```python
from build123d import *

# Parameters (mm, degrees)
F0_R         = 11.43
F0_R_2       = 14.605
F1_DEPTH     = 3.4925
F2_T1_DEPTH  = 15.875
F2_T3_DEPTH  = 15.875
F2_T5_DEPTH  = 15.875
F2_T7_DEPTH  = 15.875
F2_T10_ANGLE = 180
F2_T12_ANGLE = 90
F2_T14_ANGLE = 180
F2_T16_ANGLE = 90
F2_T18_ANGLE = 180
F2_T20_ANGLE = 90
F2_T22_ANGLE = 180
F2_T24_ANGLE = 90


# Not quite as in the source:
# - a fillet or chamfer that OpenCascade refuses, or shapes differently, is made with other operations: its cross-section is extruded or revolved along the edge and cut away or added


with BuildPart() as f1:
    # F0 (on Top) → F1 (new body)
    with BuildSketch(Plane.XY):
        with BuildLine():
            ThreePointArc((-14.605, 38.1), (0, 23.495), (14.605, 38.1))
            ThreePointArc((14.605, 38.1), (0, 52.705), (-14.605, 38.1))
        make_face()
        with Locations((0, 38.1)):
            Circle(F0_R, mode=Mode.SUBTRACT)
        with BuildLine():
            Line((14.605, 22.225), (14.605, 38.1))
            ThreePointArc((14.605, 38.1), (0, 23.495), (-14.605, 38.1))
            Line((-14.605, 38.1), (-14.605, 22.225))
            ThreePointArc((-14.605, 22.225), (-16.8368463274, 16.8368463274), (-22.225, 14.605))
            Line((-22.225, 14.605), (-38.1, 14.605))
            ThreePointArc((-38.1, 14.605), (-27.7727054608, 10.3272945392), (-23.495, 0))
            ThreePointArc((-23.495, 0), (-27.7727054608, -10.3272945392), (-38.1, -14.605))
            Line((-38.1, -14.605), (-22.225, -14.605))
            ThreePointArc((-22.225, -14.605), (-16.8368463274, -16.8368463274), (-14.605, -22.225))
            Line((-14.605, -22.225), (-14.605, -38.1))
            ThreePointArc((-14.605, -38.1), (0, -23.495), (14.605, -38.1))
            Line((14.605, -38.1), (14.605, -22.225))
            ThreePointArc((14.605, -22.225), (16.8368463274, -16.8368463274), (22.225, -14.605))
            Line((22.225, -14.605), (38.1, -14.605))
            ThreePointArc((38.1, -14.605), (23.495, 0), (38.1, 14.605))
            Line((38.1, 14.605), (22.225, 14.605))
            ThreePointArc((22.225, 14.605), (16.8368463274, 16.8368463274), (14.605, 22.225))
        make_face()
        Circle(F0_R_2, mode=Mode.SUBTRACT)
        with BuildLine():
            ThreePointArc((52.705, 0), (48.4272945392, 10.3272945392), (38.1, 14.605))
            ThreePointArc((38.1, 14.605), (23.495, 0), (38.1, -14.605))
            ThreePointArc((38.1, -14.605), (48.4272945392, -10.3272945392), (52.705, 0))
        make_face()
        with Locations((38.1, 0)):
            Circle(F0_R, mode=Mode.SUBTRACT)
        with BuildLine():
            ThreePointArc((-23.495, 0), (-27.7727054608, 10.3272945392), (-38.1, 14.605))
            ThreePointArc((-38.1, 14.605), (-52.705, 0), (-38.1, -14.605))
            ThreePointArc((-38.1, -14.605), (-27.7727054608, -10.3272945392), (-23.495, 0))
        make_face()
        with Locations((-38.1, 0)):
            Circle(F0_R, mode=Mode.SUBTRACT)
        with BuildLine():
            ThreePointArc((-14.605, -38.1), (0, -52.705), (14.605, -38.1))
            ThreePointArc((14.605, -38.1), (0, -23.495), (-14.605, -38.1))
        make_face()
        with Locations((0, -38.1)):
            Circle(F0_R, mode=Mode.SUBTRACT)
        Circle(F0_R_2)
        Circle(F0_R, mode=Mode.SUBTRACT)
    extrude(amount=F1_DEPTH)

    # F2: fillet of radius 5.08 on 1 edges, made by hand

    # F2_s2 → F2_t1 (cut)
    with BuildSketch(Plane.XZ.offset(22.225)):
        with BuildLine():
            ThreePointArc((-14.605, 0), (-12.7578317887, 2.5277703435), (-9.7794177812, 3.4925))
            Line((-9.7794177812, 3.4925), (-14.605, 3.4925))
            Line((-14.605, 3.4925), (-14.605, 0))
        make_face()
        with BuildLine():
            ThreePointArc((14.605, 0), (12.7578317887, 2.5277703435), (9.7794177812, 3.4925))
            Line((9.7794177812, 3.4925), (14.605, 3.4925))
            Line((14.605, 3.4925), (14.605, 0))
        make_face()
    extrude(amount=F2_T1_DEPTH, mode=Mode.SUBTRACT)

    # F2_s4 → F2_t3 (cut)
    with BuildSketch(Plane.YZ.offset(22.225)):
        with BuildLine():
            ThreePointArc((-14.605, 0), (-12.7578317887, 2.5277703435), (-9.7794177812, 3.4925))
            Line((-9.7794177812, 3.4925), (-14.605, 3.4925))
            Line((-14.605, 3.4925), (-14.605, 0))
        make_face()
        with BuildLine():
            ThreePointArc((14.605, 0), (12.7578317887, 2.5277703435), (9.7794177812, 3.4925))
            Line((9.7794177812, 3.4925), (14.605, 3.4925))
            Line((14.605, 3.4925), (14.605, 0))
        make_face()
    extrude(amount=F2_T3_DEPTH, mode=Mode.SUBTRACT)

    # F2_s6 → F2_t5 (cut)
    with BuildSketch(Plane.XZ.offset(-38.1)):
        with BuildLine():
            ThreePointArc((14.605, 0), (12.7578317887, 2.5277703435), (9.7794177812, 3.4925))
            Line((9.7794177812, 3.4925), (14.605, 3.4925))
            Line((14.605, 3.4925), (14.605, 0))
        make_face()
        with BuildLine():
            ThreePointArc((-14.605, 0), (-12.7578317887, 2.5277703435), (-9.7794177812, 3.4925))
            Line((-9.7794177812, 3.4925), (-14.605, 3.4925))
            Line((-14.605, 3.4925), (-14.605, 0))
        make_face()
    extrude(amount=F2_T5_DEPTH, mode=Mode.SUBTRACT)

    # F2_s8 → F2_t7 (cut)
    with BuildSketch(Plane.YZ.offset(-38.1)):
        with BuildLine():
            ThreePointArc((14.605, 0), (12.7578317887, 2.5277703435), (9.7794177812, 3.4925))
            Line((9.7794177812, 3.4925), (14.605, 3.4925))
            Line((14.605, 3.4925), (14.605, 0))
        make_face()
        with BuildLine():
            ThreePointArc((-14.605, 0), (-12.7578317887, 2.5277703435), (-9.7794177812, 3.4925))
            Line((-9.7794177812, 3.4925), (-14.605, 3.4925))
            Line((-14.605, 3.4925), (-14.605, 0))
        make_face()
    extrude(amount=F2_T7_DEPTH, mode=Mode.SUBTRACT)

    # F2_s9 → F2_t10 (revolve, cut)
    with BuildSketch(Plane.XZ.offset(38.1)):
        with BuildLine():
            ThreePointArc((-14.605, 0), (-12.7578317887, 2.5277703435), (-9.7794177812, 3.4925))
            Line((-9.7794177812, 3.4925), (-14.605, 3.4925))
            Line((-14.605, 3.4925), (-14.605, 0))
        make_face()
    revolve(axis=Axis((0, -38.1, 3.4925), (0, 0, 1)), revolution_arc=F2_T10_ANGLE, mode=Mode.SUBTRACT)

    # F2_s11 → F2_t12 (revolve, cut)
    with BuildSketch(Plane.XZ.offset(22.225)):
        with BuildLine():
            ThreePointArc((14.605, 0), (12.7578317887, 2.5277703435), (9.7794177812, 3.4925))
            Line((9.7794177812, 3.4925), (14.605, 3.4925))
            Line((14.605, 3.4925), (14.605, 0))
        make_face()
    revolve(axis=Axis((22.225, -22.225, 3.4925), (0, 0, -1)), revolution_arc=F2_T12_ANGLE, mode=Mode.SUBTRACT)

    # F2_s13 → F2_t14 (revolve, cut)
    with BuildSketch(Plane.YZ.offset(38.1)):
        with BuildLine():
            ThreePointArc((-14.605, 0), (-12.7578317887, 2.5277703435), (-9.7794177812, 3.4925))
            Line((-9.7794177812, 3.4925), (-14.605, 3.4925))
            Line((-14.605, 3.4925), (-14.605, 0))
        make_face()
    revolve(axis=Axis((38.1, 0, 3.4925), (0, 0, 1)), revolution_arc=F2_T14_ANGLE, mode=Mode.SUBTRACT)

    # F2_s15 → F2_t16 (revolve, cut)
    with BuildSketch(Plane.YZ.offset(22.225)):
        with BuildLine():
            ThreePointArc((14.605, 0), (12.7578317887, 2.5277703435), (9.7794177812, 3.4925))
            Line((9.7794177812, 3.4925), (14.605, 3.4925))
            Line((14.605, 3.4925), (14.605, 0))
        make_face()
    revolve(axis=Axis((22.225, 22.225, 3.4925), (0, 0, -1)), revolution_arc=F2_T16_ANGLE, mode=Mode.SUBTRACT)

    # F2_s17 → F2_t18 (revolve, cut)
    with BuildSketch(Plane.XZ.offset(-38.1)):
        with BuildLine():
            ThreePointArc((14.605, 0), (12.7578317887, 2.5277703435), (9.7794177812, 3.4925))
            Line((9.7794177812, 3.4925), (14.605, 3.4925))
            Line((14.605, 3.4925), (14.605, 0))
        make_face()
    revolve(axis=Axis((0, 38.1, 3.4925), (0, 0, 1)), revolution_arc=F2_T18_ANGLE, mode=Mode.SUBTRACT)

    # F2_s19 → F2_t20 (revolve, cut)
    with BuildSketch(Plane.XZ.offset(-22.225)):
        with BuildLine():
            ThreePointArc((-14.605, 0), (-12.7578317887, 2.5277703435), (-9.7794177812, 3.4925))
            Line((-9.7794177812, 3.4925), (-14.605, 3.4925))
            Line((-14.605, 3.4925), (-14.605, 0))
        make_face()
    revolve(axis=Axis((-22.225, 22.225, 3.4925), (0, 0, -1)), revolution_arc=F2_T20_ANGLE, mode=Mode.SUBTRACT)

    # F2_s21 → F2_t22 (revolve, cut)
    with BuildSketch(Plane.YZ.offset(-38.1)):
        with BuildLine():
            ThreePointArc((14.605, 0), (12.7578317887, 2.5277703435), (9.7794177812, 3.4925))
            Line((9.7794177812, 3.4925), (14.605, 3.4925))
            Line((14.605, 3.4925), (14.605, 0))
        make_face()
    revolve(axis=Axis((-38.1, 0, 3.4925), (0, 0, 1)), revolution_arc=F2_T22_ANGLE, mode=Mode.SUBTRACT)

    # F2_s23 → F2_t24 (revolve, cut)
    with BuildSketch(Plane.YZ.offset(-22.225)):
        with BuildLine():
            ThreePointArc((-14.605, 0), (-12.7578317887, 2.5277703435), (-9.7794177812, 3.4925))
            Line((-9.7794177812, 3.4925), (-14.605, 3.4925))
            Line((-14.605, 3.4925), (-14.605, 0))
        make_face()
    revolve(axis=Axis((-22.225, -22.225, 3.4925), (0, 0, -1)), revolution_arc=F2_T24_ANGLE, mode=Mode.SUBTRACT)


solid = f1.part
```
Verification items for the finished model (mm, model axes). A direction names the side the tool comes from. Coordinates: 2 decimals unless noted, no trailing zeros. Order: outer loops, then holes, each group sorted by start corner. A loop starts at its lowest first (then second) coordinate and runs counter-clockwise, first axis right, second up. Notation, with made-up numbers: (89, -19.75) - (143, -19.75) arc R25 cw to (143, 14.25) - close; hole circle Ø6 at (48, 32.5). An arc over 180 degrees is marked (long way). Return JSON: item names as keys, results as strings.
(1) Section check D-D, the plane x = 24. Record the cut outline in (y, z) (1 decimal), and give its area (3 significant figures).
Filled sheet:
{"outline": "(-14.6, 0) - (14.6, 0) arc R5.1 ccw to (9.8, 3.5) - (-9.8, 3.5) arc R5.1 ccw to start", "area": "93.0 mm^2"}
(2) Section check C-C, the plane z = 1.2. Record the cut outline in (x, y) (3 decimals), and give its area (3 significant figures).
Filled sheet:
{"outline": "(-38.1, -14.026) - (-22.225, -14.026) arc R8.199 cw to (-14.026, -22.225) - (-14.026, -38.1) arc R14.026 ccw to (14.026, -38.1) - (14.026, -22.225) arc R8.199 cw to (22.225, -14.026) - (38.1, -14.026) arc R14.026 ccw to (38.1, 14.026) - (22.225, 14.026) arc R8.199 cw to (14.026, 22.225) - (14.026, 38.1) arc R14.026 ccw to (-14.026, 38.1) - (-14.026, 22.225) arc R8.199 cw to (-22.225, 14.026) - (-38.1, 14.026) arc R14.026 ccw to start; hole circle Ø22.86 at (-38.1, 0); hole circle Ø22.86 at (0, -38.1); hole circle Ø22.86 at (0, 0); hole circle Ø22.86 at (0, 38.1); hole circle Ø22.86 at (38.1, 0)", "area": "2,730 mm^2"}
(3) Mould release check, pull along Y, two halves, no side actions. Record for faces 1 (the cylindrical face through (29.03, -6.955, 1.722)), 2 (the flat face through (0, 12, 0)), 3 (the cylindrical face through (-30.274, -12.794, 2.501)): pulls with the +Y half, pulls with the -Y half, needs draft (parallel to the pull), parting line crosses it, or undercut.
Filled sheet:
{"face 1": "undercut", "face 2": "needs draft", "face 3": "pulls with the -Y half"}
(4) Go/stop test with flat-tipped pins: pin 1 (6 mm diameter, centred on x = -18.5, y = -36, fed in from -Z); pin 2 (2 mm diameter, centred on x = 11.5, z = 1.5, fed in from -Y). Record where each tip stops, or that it passes through.
Filled sheet:
{"pin 1": "passes through", "pin 2": "stops at y = -47.45"}
(5) Access from +Z, -Z, +X, -X, +Y, -Y to the whole of each face (thin tool, end or side, straight path). Record for faces 4 (the cylindrical face through (-12.794, -30.051, 2.501)), 5 (the cylindrical face through (12.794, -30.051, 2.501)), 6 (the cylindrical face through (-12.794, 30.274, 2.501)), 7 (the cylindrical face through (10.902, 3.433, 1.722)), 8 (the cylindrical face through (12.794, 30.274, 2.501)).
Filled sheet:
{"face 4": "+Z, -X, -Y", "face 5": "+Z, +X, -Y", "face 6": "+Z, -X, +Y", "face 7": "+Z, -Z", "face 8": "+Z, +X, +Y"}
(6) Thickness scan on line 1 along Y through (x, z) = (0, 2.05); line 2 along Y through (x, z) = (0, 1.3); line 3 along X through (y, z) = (3.5, 1.75). Record the ranges inside material, lowest first.
Filled sheet:
{"line 1": "y = -51.43 to -49.53, -26.67 to -11.43, 11.43 to 26.67, 49.53 to 51.43", "line 2": "y = -52.06 to -49.53, -26.67 to -11.43, 11.43 to 26.67, 49.53 to 52.06", "line 3": "x = -51.25 to -48.98, -27.22 to -10.88, 10.88 to 27.22, 48.98 to 51.25"}
(7) Section check A-A, the plane x = 0. Record the cut outline in (y, z) (1 decimal).
Filled sheet:
{"outline": "(-52.7, 0) - (-49.5, 0) - (-49.5, 3.2) arc R5.1 ccw to start; (-26.7, 0) - (-11.4, 0) - (-11.4, 3.5) - (-26.7, 3.5) - close; (11.4, 0) - (26.7, 0) - (26.7, 3.5) - (11.4, 3.5) - close; (49.5, 0) - (52.7, 0) arc R5.1 ccw to (49.5, 3.2) - close"}
